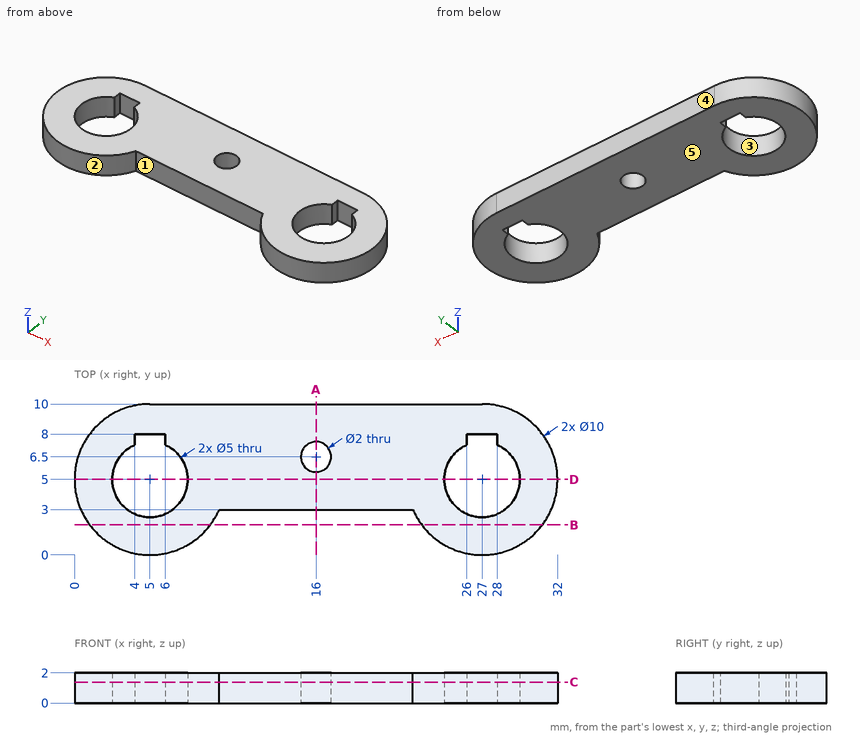
Geometry: see drawing. Coordinates: mm, zero at the bounding-box minimum. A direction names the side the tool comes from. Round coordinates to 2 decimals unless told otherwise and drop trailing zeros. Loops run counter-clockwise (first coordinate to the right, second up) from the corner with the lowest first, then second, coordinate; pieces in that order, holes last. Notation, with made-up numbers: (69, 22) - (74, 22) arc R25 ccw to (74, 57) - close; hole circle Ø9 at (74, -9.5). An arc over 180 degrees is marked (long way). Write item = value, one per line. Start each with the question number.
(1) Pull-direction query (Y, two-part tool) for the marked faces 3, 4 and 5; classes: +Y half, -Y half, draft (parallel to the pull), parting line (faces both ways), or undercut.
(2) Section query B-B, the plane y = 2. Output: boundary loops of the cut face in (x, z).
(3) Ray query, line 1 along X through (y, z) = (5, 1.1); line 2 along Y through (x, z) = (16, 0.6); line 3 along X through (y, z) = (4.5, 1.1). Return the intervals inside material, ascending. Write a range as from..to.
(4) Section query D-D, the plane y = 5. Output: boundary loops of the cut face in (x, z), plus the area to 3 significant figures.
(5) Section query C-C, the plane z = 1.4. Output: boundary loops of the cut face in (x, y), plus the area to 3 significant figures.
(6) Section query A-A, the plane x = 16. Output: boundary loops of the cut face in (y, z).
(7) Set-up query: the marked faces 1 and 2. Return all of +Z, -Z, +X, -X, +Y, -Y with unobstructed straight access to the full face (end or side cutting, diameter ignored); none if empty.
Conclusion:
q1.face_3 = undercut
q1.face_4 = +Y half
q1.face_5 = draft
q2.outline = (1, 0) - (9, 0) - (9, 2) - (1, 2) - close; (23, 0) - (31, 0) - (31, 2) - (23, 2) - close
q3.line_1 = 0..2.5, 7.5..24.5, 29.5..32
q3.line_2 = 3..5.5, 7.5..10
q3.line_3 = 0.03..2.55, 7.45..24.55, 29.45..31.97
q4.outline = (0, 0) - (2.5, 0) - (2.5, 2) - (0, 2) - close; (7.5, 0) - (24.5, 0) - (24.5, 2) - (7.5, 2) - close; (29.5, 0) - (32, 0) - (32, 2) - (29.5, 2) - close
q4.area = 44.0 mm2
q5.outline = (5, 10) arc R5 ccw (long way) to (9.58, 3) - (22.42, 3) arc R5 ccw (long way) to (27, 10) - close; hole (4, 7.29) arc R2.5 ccw (long way) to (6, 7.29) - (6, 8) - (4, 8) - close; hole circle Ø2 at (16, 6.5); hole (26, 7.29) arc R2.5 ccw (long way) to (28, 7.29) - (28, 8) - (26, 8) - close
q5.area = 208 mm2
q6.outline = (3, 0) - (5.5, 0) - (5.5, 2) - (3, 2) - close; (7.5, 0) - (10, 0) - (10, 2) - (7.5, 2) - close
q7.face_1 = +Z, -Z, -Y
q7.face_2 = +Z, -Z
